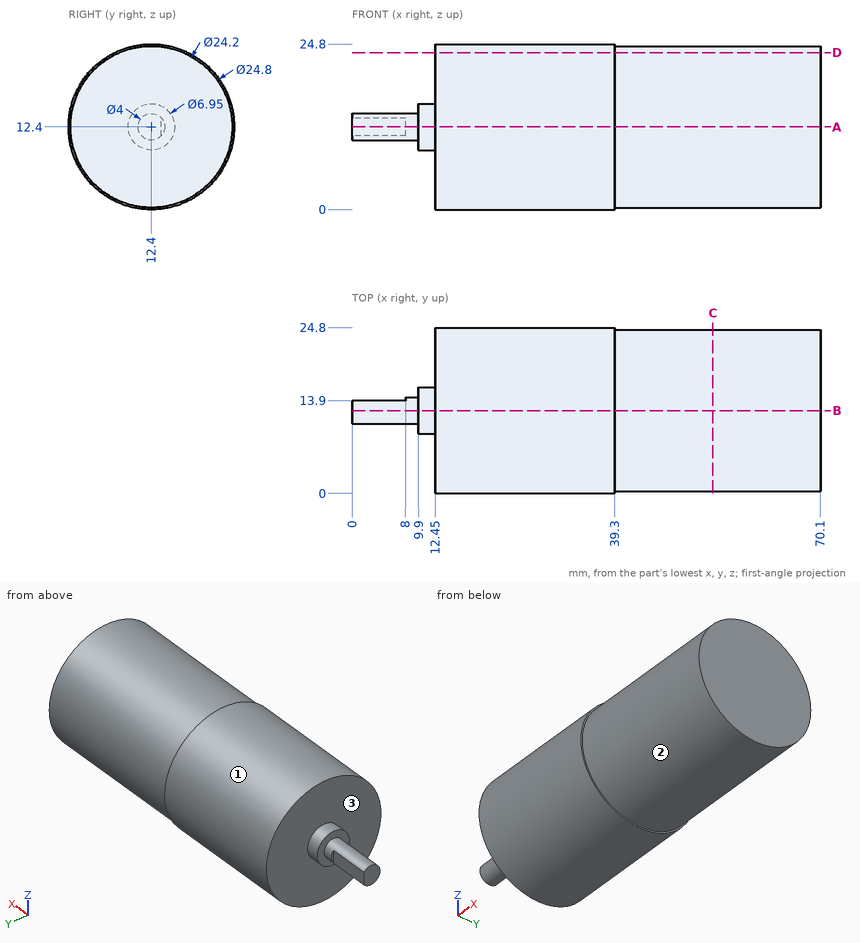
Part print with two shaded views. Sizes in mm from the minimum x, y, z corner. A direction names the side the tool comes from. Round coordinates to 2 decimals unless told otherwise and drop trailing zeros. Loops run counter-clockwise (first coordinate to the right, second up) from the corner with the lowest first, then second, coordinate; pieces in that order, holes last.
Item 1: Which spindle directions (+Z, -Z, +X, -X, +Y, -Y) get a long thin tool onto all of the face, cutting with end or side? Do the marked faces 1, 2 and 3. Say none if no direction does.
Item 2: Pin check, flat tips, straight feed: P1, Ø3, axis at x = 3.5, z = 12.5, coming from the +Y side; P2, Ø1, axis at y = 17.5, z = 13, coming from the -X side; P3, Ø1.5, axis at x = 49.5, y = 10.5, coming from the +Z side; P4, Ø5.5, axis at y = 13, z = 11.5, coming from the -X side. Stop position of each tip, or through.
Item 3: Saw through at A-A (z = 12.4). List the corners of the cut face in (x, y) (3 decimals), then the cut area to 3 significant figures.
Item 4: Saw through at B-B (y = 12.4). List the corners of the cut face in (x, z) (3 decimals), then the cut area to 3 significant figures.
Item 5: Drill centre lines: line 1 along X through (y, z) = (13, 8.25); line 2 along Y through (x, z) = (49.5, 6); line 3 along Y through (x, z) = (55, 12.75). Where is each one in solid material? Low to high.
Item 6: Saw through at C-C (x = 54). List the corners of the cut face in (y, z), then the cut area to 3 significant figures.
Item 7: Saw through at D-D (z = 23.5). List the corners of the cut face in (x, y), then the cut area to 3 significant figures.
Worked answers:
1. face 1: +X, -X
1. face 2: +X
1. face 3: -X
2. P1: stops at y = 13.9
2. P2: stops at x = 12.45
2. P3: stops at z = 24.45
2. P4: stops at x = 0
3. outline: (0, 10.4) - (9.9, 10.4) - (9.9, 8.925) - (12.45, 8.925) - (12.45, 0) - (39.3, 0) - (39.3, 0.3) - (70.1, 0.3) - (70.1, 24.5) - (39.3, 24.5) - (39.3, 24.8) - (12.45, 24.8) - (12.45, 15.875) - (9.9, 15.875) - (9.9, 14.4) - (8, 14.4) - (8, 13.9) - (0, 13.9) - close
3. area: 1,460 mm2
4. outline: (0, 10.4) - (9.9, 10.4) - (9.9, 8.925) - (12.45, 8.925) - (12.45, 0) - (39.3, 0) - (39.3, 0.3) - (70.1, 0.3) - (70.1, 24.5) - (39.3, 24.5) - (39.3, 24.8) - (12.45, 24.8) - (12.45, 15.875) - (9.9, 15.875) - (9.9, 14.4) - (0, 14.4) - close
4. area: 1,470 mm2
5. line 1: x = 12.45 to 70.1
5. line 2: y = 2.13 to 22.67
5. line 3: y = 0.31 to 24.49
6. outline: circle Ø24.2 at (12.4, 12.4)
6. area: 460 mm2
7. outline: (12.45, 6.87) - (39.3, 6.87) - (39.3, 7.58) - (70.1, 7.58) - (70.1, 17.22) - (39.3, 17.22) - (39.3, 17.93) - (12.45, 17.93) - close
7. area: 594 mm2
